Source: CAD feature listing. Evaluate the final solid. Frame: model axes, mm. Face numbers are marked on the shaded views. A direction names the side the tool comes from. Round coordinates to 2 decimals unless told otherwise and drop trailing zeros. Loops run counter-clockwise (first coordinate to the right, second up) from the corner with the lowest first, then second, coordinate; pieces in that order, holes last. Notation, with made-up numbers: (-37, 53) - (16, 53) arc R8 cw to (16, 60) - close; hole circle Ø7 at (64.25, 9). An arc over 180 degrees is marked (long way). Use CSV: the item, a comma, the result in double quotes. Start each with the question number.
from build123d import *

# Parameters (mm, degrees)
BOSS_EXTRUDE1_DEPTH = 12
SKETCH2_W           = 6.5
SKETCH2_H           = 6
CUT_EXTRUDE1_DEPTH  = 36.003571246
SKETCH3_R           = 1.5
CUT_EXTRUDE2_DEPTH  = 12
SKETCH6_R           = 1.5
CUT_EXTRUDE3_DEPTH  = 36.003571246
FILLET1_R           = 2.5


with BuildPart() as part:
    # Sketch1 → Boss-Extrude1 (new body)
    with BuildSketch(Plane.XY):
        with BuildLine():
            Line((0, 0), (30, 0))
            ThreePointArc((30, 0), (32.5, 2.5), (30, 5))
            Line((30, 5), (0, 5))
            Line((0, 5), (0, 0))
        make_face()
    extrude(amount=-BOSS_EXTRUDE1_DEPTH)

    # Sketch2 → Cut-Extrude1 (cut, through all)
    with BuildSketch(Plane(origin=(0, 5, 0), x_dir=(1, 0, 0), z_dir=(0, 1, 0))):
        with Locations((29.25, 6)):
            Rectangle(SKETCH2_W, SKETCH2_H)
    extrude(amount=-CUT_EXTRUDE1_DEPTH, mode=Mode.SUBTRACT)

    # Sketch3 → Cut-Extrude2 (cut)
    with BuildSketch(Plane.XY):
        with Locations((30, 2.5)):
            Circle(SKETCH3_R)
    extrude(amount=-CUT_EXTRUDE2_DEPTH, mode=Mode.SUBTRACT)

    # Sketch6 → Cut-Extrude3 (cut, through all)
    with BuildSketch(Plane(origin=(0, 5, 0), x_dir=(1, 0, 0), z_dir=(0, 1, 0))):
        with Locations(Location((3, 6, 0), (0, 0, 270))):
            Circle(SKETCH6_R)
    extrude(amount=-CUT_EXTRUDE3_DEPTH, mode=Mode.SUBTRACT)

    # Fillet1
    fillet1_edges = [part.edges().sort_by_distance(p)[0] for p in [
        (0, 2.5, -12),
        (0, 2.5, 0),
    ]]
    fillet(fillet1_edges, radius=FILLET1_R)


solid = part.part
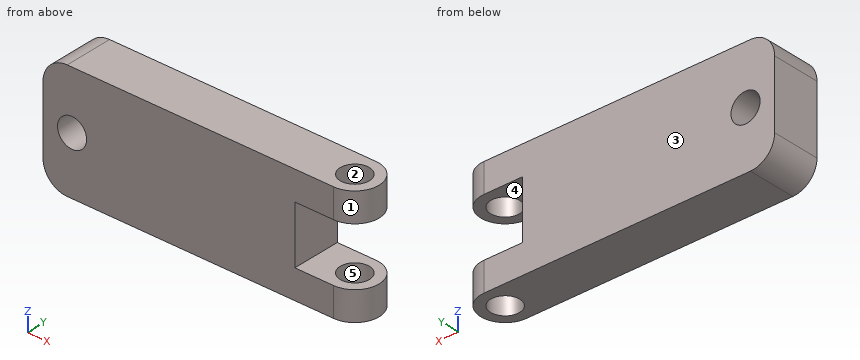
1. Section query C-C on y = 4.4. Return the cut outline in (x, z).
2. Contact query for a flat-ended pin moving along its axis: P1, Ø1, axis at y = 3.5, z = -1, coming from the +X side. Output: stop coordinate, or through.
3. Mould query, pull axis X, two halves, no side actions, for the marked faces 1, 2 and 3. Classes: +X half, -X half, draft (parallel to the pull), parting line (faces both ways), or undercut.
4. Reachability of the marked faces 4 and 5 from +Z, -Z, +X, -X, +Y, -Y: full face, straight path, thin tool, end or side. Return the list, or none.
5. Section query A-A on x = 28. Return the cut outline in (y, z).
6. Line query: line 1 along Y through (x, z) = (30, -9.7); line 2 along Z through (x, y) = (27.5, 1.2); line 3 along X through (y, z) = (1.9, -6). Output: solid intervals per line, ascending.
7. Section query B-B on z = -6. Return the cut outline in (x, y).
8. Section query D-D on z = -10.5. Return the cut outline in (x, y), and give its area (3 significant figures).
Values:
1,outline,"(0, -9.5) arc R2.5 ccw to (2.5, -12) - (31.62, -12) - (31.62, -9) - (26, -9) - (26, -3) - (31.62, -3) - (31.62, 0) - (2.5, 0) arc R2.5 ccw to (0, -2.5) - close; hole circle Ø3 at (3, -6)"
2,P1,"stops at x = 32.45"
3,face 1,"+X half"
3,face 2,"undercut"
3,face 3,"draft"
4,face 4,"+X, +Y, -Y"
4,face 5,"+Z, -Z"
5,outline,"(0, -12) - (5, -12) - (5, -9) - (0, -9) - close; (0, -3) - (5, -3) - (5, 0) - (0, 0) - close"
6,line 1,"y = 0 to 1, 4 to 5"
6,line 2,"z = -12 to -9, -3 to 0"
6,line 3,"x = 0 to 1.5, 4.5 to 26"
7,outline,"(0, 0) - (1.5, 0) - (1.5, 5) - (0, 5) - close; (4.5, 0) - (26, 0) - (26, 5) - (4.5, 5) - close"
8,outline,"(0.21, 0) - (30, 0) arc R2.5 ccw to (30, 5) - (0.21, 5) - close; hole circle Ø3 at (30, 2.5)"
8,area,"152 mm^2"
